Geometry check sheet. Reference: the model listing, model coordinates, mm. A direction names the side the tool comes from. Coordinates: 2 decimals unless noted, no trailing zeros. Loops run counter-clockwise (first coordinate to the right, second up) from the corner with the lowest first, then second, coordinate; pieces in that order, holes last. Notation, with made-up numbers: (84.25, 11.5) -> (88.25, 11.5) arc R28 ccw to (88.25, 34.5) -> close; hole circle Ø5 at (7.5, 82). An arc over 180 degrees is marked (long way). Answer as a JSON object with one key per item and string values.
Autodesk Inventor part; units mm, degrees
sketch "Esboço1" plane through (0, 0, 0) normal (1, 0, 0) x (0, 1, 0)
  line L0 (-340, -390) -> (340, -390)
  line L1 (375, -355) -> (375, 355)
  line L2 (340, 390) -> (-340, 390)
  line L3 (-375, 355) -> (-375, -355)
  line L4 (-375, -390) -> (375, 390) construction
  line L5 (375, -390) -> (-375, 390) construction
  line L6 (-310, -358.8) -> (310, -358.8)
  line L7 (345, -323.8) -> (345, 323.8)
  line L8 (310, 358.8) -> (-310, 358.8)
  line L9 (-345, 323.8) -> (-345, -323.8)
  line L10 (-345, -358.8) -> (345, 358.8) construction
  line L11 (345, -358.8) -> (-345, 358.8) construction
  arc A0 (345, 323.8) -> (310, 358.8) centre (310, 323.8) ccw
  arc A1 (375, 355) -> (340, 390) centre (340, 355) ccw
  arc A2 (340, -390) -> (375, -355) centre (340, -355) ccw
  arc A3 (310, -358.8) -> (345, -323.8) centre (310, -323.8) ccw
  arc A4 (-310, 358.8) -> (-345, 323.8) centre (-310, 323.8) ccw
  arc A5 (-345, -323.8) -> (-310, -358.8) centre (-310, -323.8) ccw
  arc A6 (-375, -355) -> (-340, -390) centre (-340, -355) ccw
  arc A7 (-340, 390) -> (-375, 355) centre (-340, 355) ccw
  point P0 (0, 0)
  dimension "d0" = 780
  dimension "d1" = 750
  dimension "d2" = 30
  dimension "d3" = 35
  dimension "d4" = 35
  dimension "d5" = 35
extrude "Extrusão1" add sketch "Esboço1" along normal mid plane 30
equation "\"Raio_vergadura\" = Espessura"
equation "\"Largura_alívio_de_vergadura\" = Espessura"
equation "\"Profundidade_alívio_de_vergadura\" = 0.5 * Espessura"
equation "\"Tamanho_alívio_de_dobra\" = 4 * Espessura"
equation "\"Remanescente_mínimo\" = 2 * Espessura"
equation "\"Raiodetransição\" = Raio_vergadura"
equation "\"Tamanho_de_raio_de_Jacobi\" = Raio_vergadura"
equation "\"TamanhoFolga\" = Espessura"
properties part number "Pés"
1. Section check B-B, the plane z = 144.5. Record the boundary of the cut face in (x, y).
Evaluation:
{"outline": "(-15, -375) -> (15, -375) -> (15, -345) -> (-15, -345) -> close; (-15, 345) -> (15, 345) -> (15, 375) -> (-15, 375) -> close"}
2. Section check A-A, the plane y = 106. Record the boundary of the cut face in (x, z), then the cut area to 3 significant figures.
Evaluation:
{"outline": "(-15, -390) -> (15, -390) -> (15, -358.8) -> (-15, -358.8) -> close; (-15, 358.8) -> (15, 358.8) -> (15, 390) -> (-15, 390) -> close", "area": "1,870 mm^2"}
3. Thickness scan on probe 1 along Y at (x, z) = (-1, 131); probe 2 along Z at (x, y) = (-3.5, -281.5); probe 3 along Y at (x, z) = (-9.5, 355). Record the ranges inside material, lowest first. Write a range as from..to.
Evaluation:
{"probe 1": "y = -375..-345, 345..375", "probe 2": "z = -390..-358.8, 358.8..390", "probe 3": "y = -375..-325.86, 325.86..375"}
4. Section check C-C, the plane x = 6.5. Record the boundary of the cut face in (y, z).
Evaluation:
{"outline": "(-375, -355) arc R35 ccw to (-340, -390) -> (340, -390) arc R35 ccw to (375, -355) -> (375, 355) arc R35 ccw to (340, 390) -> (-340, 390) arc R35 ccw to (-375, 355) -> close; hole (-345, -323.8) arc R35 ccw to (-310, -358.8) -> (310, -358.8) arc R35 ccw to (345, -323.8) -> (345, 323.8) arc R35 ccw to (310, 358.8) -> (-310, 358.8) arc R35 ccw to (-345, 323.8) -> close"}
5. Mould release check, pull along Y, two halves, no side actions. Record for faces 1 (the face through (0, -345, 5)), 2 (the face through (-0.21, -365.019, 379.475)), 3 (the face through (0, -5, -390)): released by +Y, released by -Y, zero draft, split by the parting line, or undercut.
Evaluation:
{"face 1": "undercut", "face 2": "released by -Y", "face 3": "zero draft"}
6. Tool access check on faces 4 (the face through (-0.21, 334.475, 348.819)), 5 (the face through (0, 375, -5)). Record the directions out of +Z, -Z, +X, -X, +Y, -Y that give a thin tool (end or side, any length) a straight path to the whole face; none if there is none.
Evaluation:
{"face 4": "+X, -X", "face 5": "+Z, -Z, +X, -X, +Y"}
